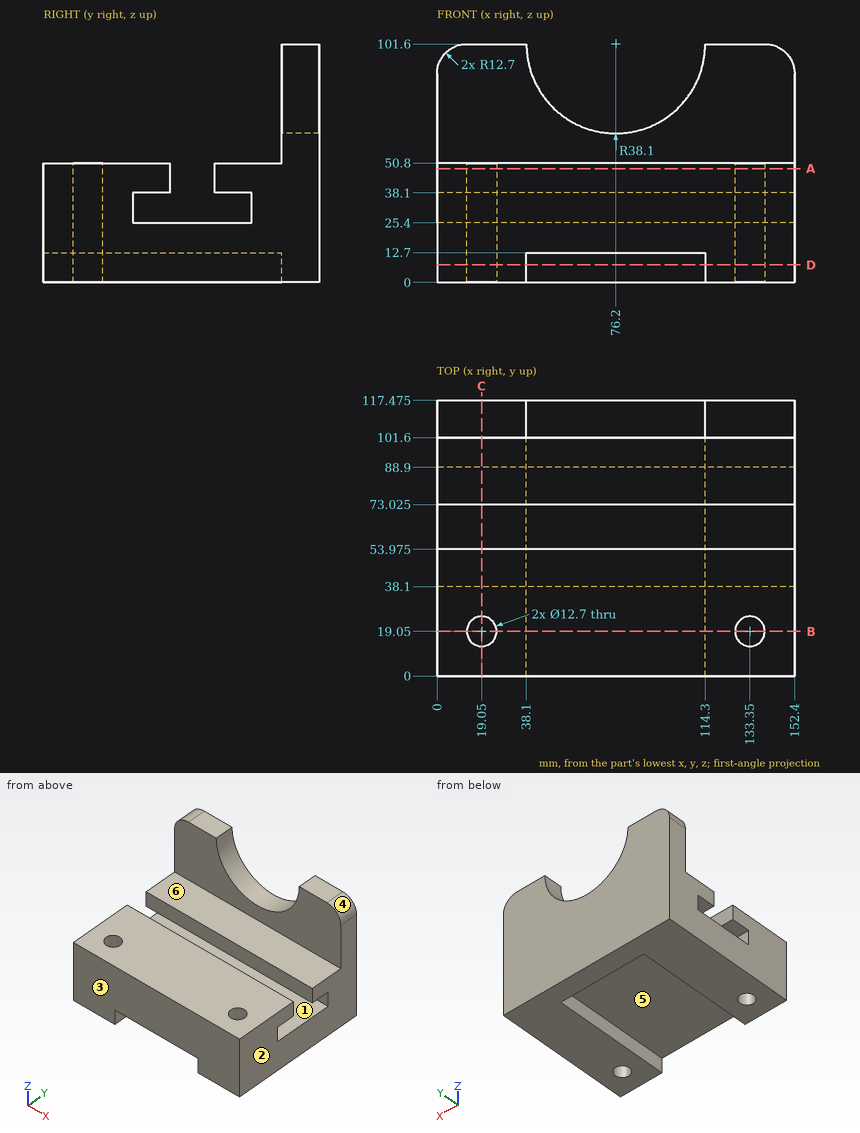
Check sheet for the drawn part. Datum: minimum x, y, z corner. Units: mm. A direction names the side the tool comes from. Coordinates: 2 decimals unless noted, no trailing zeros. Write each loop counter-clockwise with the first axis right and the second up, starting at its lowest first coordinate (ties: lowest second). Pieces come first, ordered by that corner, then holes. Notation, with made-up numbers: (22, 4) - (50, 4) arc R23 ccw to (50, 43) - close; hole circle Ø10 at (29, 46.5). An arc over 180 degrees is marked (long way). Answer as a JSON object with one key per item and string values.
(1) Cross-section at B-B on y = 19.05. Record the cut outline in (x, z), plus the area to 3 significant figures.
Report:
{"outline": "(0, 0) - (12.7, 0) - (12.7, 50.8) - (0, 50.8) - close; (25.4, 0) - (38.1, 0) - (38.1, 12.7) - (114.3, 12.7) - (114.3, 0) - (127, 0) - (127, 50.8) - (25.4, 50.8) - close; (139.7, 0) - (152.4, 0) - (152.4, 50.8) - (139.7, 50.8) - close", "area": "5,480 mm^2"}
(2) Cross-section at D-D on z = 7.5. Record the cut outline in (x, y) (3 decimals), plus the area to 3 significant figures.
Report:
{"outline": "(0, 0) - (38.1, 0) - (38.1, 101.6) - (114.3, 101.6) - (114.3, 0) - (152.4, 0) - (152.4, 117.475) - (0, 117.475) - close; hole circle Ø12.7 at (19.05, 19.05); hole circle Ø12.7 at (133.35, 19.05)", "area": "9,910 mm^2"}
(3) Gauge pin test, flat ends, axial feed: pin 1 Ø10 at (x, y) = (133.35, 19.05) entering from +Z; pin 2 Ø1.5 at (x, y) = (39, 44.5) entering from -Z; pin 3 Ø23 at (x, y) = (86.5, 88) entering from +Z; pin 4 Ø15 at (x, z) = (101, 83) entering from -Y. Record the tip position at first contact, or that the pin passes through.
Report:
{"pin 1": "through", "pin 2": "z = 12.7", "pin 3": "z = 50.8", "pin 4": "y = 101.6"}
(4) Thickness scan on line 1 along X through (y, z) = (19, 34); line 2 along Y through (x, z) = (133, 36) (3 decimals); line 3 along Y through (x, z) = (133, 11) (3 decimals). Record the ranges inside material, lowest first.
Report:
{"line 1": "0 to 12.7, 25.4 to 127, 139.7 to 152.4", "line 2": "0 to 12.71, 25.39 to 38.1, 88.9 to 117.475", "line 3": "0 to 12.71, 25.39 to 117.475"}
(5) Cross-section at A-A on z = 48.5. Record the cut outline in (x, y) (3 decimals), plus the area to 3 significant figures.
Report:
{"outline": "(0, 0) - (152.4, 0) - (152.4, 53.975) - (0, 53.975) - close; (0, 73.025) - (152.4, 73.025) - (152.4, 117.475) - (0, 117.475) - close; hole circle Ø12.7 at (19.05, 19.05); hole circle Ø12.7 at (133.35, 19.05)", "area": "14,700 mm^2"}
(6) Tool access check on the marked faces 4, 5 and 6. Record the directions out of +Z, -Z, +X, -X, +Y, -Y that give a thin tool (end or side, any length) a straight path to the whole face; none if there is none.
Report:
{"face 4": "+Z, +X, +Y, -Y", "face 5": "-Z, -Y", "face 6": "+Z, +X, -X, -Y"}
(7) Cross-section at C-C on x = 19.05. Record the cut outline in (y, z) (3 decimals).
Report:
{"outline": "(0, 0) - (12.7, 0) - (12.7, 50.8) - (0, 50.8) - close; (25.4, 0) - (117.475, 0) - (117.475, 101.6) - (101.6, 101.6) - (101.6, 50.8) - (73.025, 50.8) - (73.025, 38.1) - (88.9, 38.1) - (88.9, 25.4) - (38.1, 25.4) - (38.1, 38.1) - (53.975, 38.1) - (53.975, 50.8) - (25.4, 50.8) - close"}
(8) Mould release check, pull along Y, two halves, no side actions. Record for the marked faces 1, 2 and 3: pulls with the +Y half, pulls with the -Y half, needs draft (parallel to the pull), parting line crosses it, or undercut.
Report:
{"face 1": "undercut", "face 2": "needs draft", "face 3": "pulls with the -Y half"}
